from build123d import *

# Parameters (mm, degrees)
SKETCH1_R           = 25
SKETCH1_R_2         = 5
BOSS_EXTRUDE1_DEPTH = 15
SKETCH2_R           = 5
CUT_EXTRUDE1_DEPTH  = 39.405728739


with BuildPart() as part:
    # Sketch1 → Boss-Extrude1 (new body)
    with BuildSketch(Plane(origin=(0, 0, 0), x_dir=(1, 0, 0), z_dir=(0, 1, 0))):
        with Locations(Location((0, 0, 0), (0, 0, 270))):
            Circle(SKETCH1_R)
        with Locations(Location((10.606601718, 10.606601718, 0), (0, 0, 270))):
            Circle(SKETCH1_R_2, mode=Mode.SUBTRACT)
        with Locations(Location((10.606601718, -10.606601718, 0), (0, 0, 270))):
            Circle(SKETCH1_R_2, mode=Mode.SUBTRACT)
        with Locations(Location((-10.606601718, -10.606601718, 0), (0, 0, 270))):
            Circle(SKETCH1_R_2, mode=Mode.SUBTRACT)
        with Locations(Location((-10.606601718, 10.606601718, 0), (0, 0, 270))):
            Circle(SKETCH1_R_2, mode=Mode.SUBTRACT)
    extrude(amount=BOSS_EXTRUDE1_DEPTH)

    # Sketch2 → Cut-Extrude1 (cut, through all)
    with BuildSketch(Plane(origin=(0, 15, 0), x_dir=(1, 0, 0), z_dir=(0, 1, 0))):
        with Locations(Location((0, 0, 0), (0, 0, 270))):
            Circle(SKETCH2_R)
    extrude(amount=-CUT_EXTRUDE1_DEPTH, mode=Mode.SUBTRACT)


solid = part.part
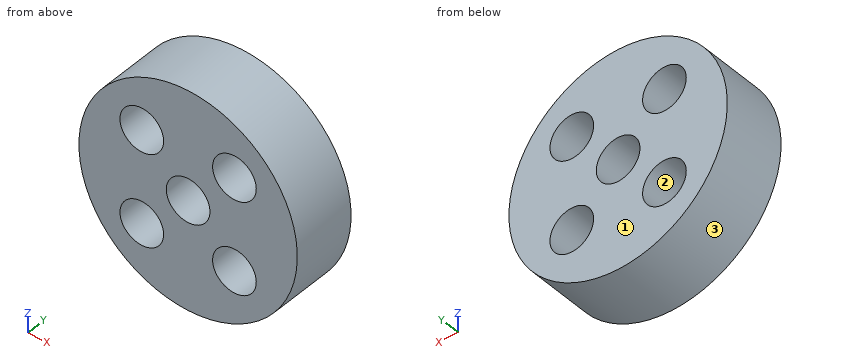
Here's how the part is built. I have some questions about the finished solid (model axes, mm). Face numbers are marked on the shaded views. Coordinates: 2 decimals unless noted, no trailing zeros. Write each loop counter-clockwise with the first axis right and the second up, starting at its lowest first coordinate (ties: lowest second). Pieces come first, ordered by that corner, then holes.
Item 1: If we mould it in two halves opening along Z, with no side actions, what happens to the marked faces 1, 2 and 3? For each: +Z half, -Z half, draft (parallel to the pull), parting line (faces both ways), or undercut.
Item 2: If I drill on line 1 (X direction, y = 8.75, z = 0); line 2 (Z direction, x = -6, y = 4.5); line 3 (Z direction, x = -13.5, y = 9.25), over which ranges is the centre line in solid material (lowest first)?
Item 3: I want a section at C-C on z = 13.5. Write out the boundary of the cut face in (x, y), and give its area (3 significant figures).
Item 4: I want a section at B-B on x = 0. Write out the boundary of the cut face in (y, z), and give its area (3 significant figures).
Item 5: I want a section at D-D on x = -14.5. Write out the boundary of the cut face in (y, z), and give its area (3 significant figures).
Item 6: Will these pins go through, and if not, where does the flat tip stop? pin 1 (8 mm diameter, centred on x = 0, z = 0, fed in from -Y); pin 2 (2 mm diameter, centred on y = 10, z = 7.5, fed in from +X); pin 3 (2 mm diameter, centred on x = 15, y = 2, fed in from -Z); pin 4 (6 mm diameter, centred on y = 13, z = -12, fed in from +X).
Item 7: I want a section at A-A on z = 0. Write out the boundary of the cut face in (x, y), and give its area (3 significant figures).
Findings below:
1. face 1: draft
1. face 2: undercut
1. face 3: parting line
2. line 1: x = -25 to -5, 5 to 25
2. line 2: z = -24.27 to -12.55, -8.66 to 8.66, 12.55 to 24.27
2. line 3: z = -21.04 to -14.68, -6.53 to 6.53, 14.68 to 21.04
3. outline: (-21.04, 0) - (-14.68, 0) - (-14.68, 15) - (-21.04, 15) - close; (-6.53, 0) - (6.53, 0) - (6.53, 15) - (-6.53, 15) - close; (14.68, 0) - (21.04, 0) - (21.04, 15) - (14.68, 15) - close
3. area: 387 mm2
4. outline: (0, -25) - (15, -25) - (15, -5) - (0, -5) - close; (0, 5) - (15, 5) - (15, 25) - (0, 25) - close
4. area: 600 mm2
5. outline: (0, -20.37) - (15, -20.37) - (15, -13.74) - (0, -13.74) - close; (0, -7.47) - (15, -7.47) - (15, 7.47) - (0, 7.47) - close; (0, 13.74) - (15, 13.74) - (15, 20.37) - (0, 20.37) - close
5. area: 423 mm2
6. pin 1: passes through
6. pin 2: stops at x = 24.14
6. pin 3: stops at z = -20.71
6. pin 4: stops at x = 23.32
7. outline: (-25, 0) - (-5, 0) - (-5, 15) - (-25, 15) - close; (5, 0) - (25, 0) - (25, 15) - (5, 15) - close
7. area: 600 mm2
